```python
from build123d import *

# Parameters (mm, degrees)
BOSS_EXTRUDE1_DEPTH = 1


with BuildPart() as part:
    # Sketch1 → Boss-Extrude1 (new body)
    with BuildSketch(Plane.XY):
        with BuildLine():
            Line((-72.995, -45.925), (-72.995, 45.925))
            ThreePointArc((-72.995, 45.925), (-71.676980515, 49.106980515), (-68.495, 50.425))
            Line((-68.495, 50.425), (61.423932188, 50.425))
            ThreePointArc((61.423932188, 50.425), (63.146007634, 50.082457896), (64.605912703, 49.106980515))
            Line((64.605912703, 49.106980515), (71.676980515, 42.035912703))
            ThreePointArc((71.676980515, 42.035912703), (72.652457896, 40.576007634), (72.995, 38.853932188))
            Line((72.995, 38.853932188), (72.995, -38.853932188))
            ThreePointArc((72.995, -38.853932188), (72.652457896, -40.576007634), (71.676980515, -42.035912703))
            Line((71.676980515, -42.035912703), (64.605912703, -49.106980515))
            ThreePointArc((64.605912703, -49.106980515), (63.146007634, -50.082457896), (61.423932188, -50.425))
            Line((61.423932188, -50.425), (-68.495, -50.425))
            ThreePointArc((-68.495, -50.425), (-71.676980515, -49.106980515), (-72.995, -45.925))
        make_face()
        with BuildLine():
            Line((-71.995, 45.925), (-71.995, -45.925))
            ThreePointArc((-71.995, -45.925), (-70.969873734, -48.399873734), (-68.495, -49.425))
            Line((-68.495, -49.425), (61.423932188, -49.425))
            ThreePointArc((61.423932188, -49.425), (62.763324201, -49.158578364), (63.898805922, -48.399873734))
            Line((63.898805922, -48.399873734), (70.969873734, -41.328805922))
            ThreePointArc((70.969873734, -41.328805922), (71.728578364, -40.193324201), (71.995, -38.853932188))
            Line((71.995, -38.853932188), (71.995, 38.853932188))
            ThreePointArc((71.995, 38.853932188), (71.728578364, 40.193324201), (70.969873734, 41.328805922))
            Line((70.969873734, 41.328805922), (63.898805922, 48.399873734))
            ThreePointArc((63.898805922, 48.399873734), (62.763324201, 49.158578364), (61.423932188, 49.425))
            Line((61.423932188, 49.425), (-68.495, 49.425))
            ThreePointArc((-68.495, 49.425), (-70.969873734, 48.399873734), (-71.995, 45.925))
        make_face(mode=Mode.SUBTRACT)
    extrude(amount=BOSS_EXTRUDE1_DEPTH)


solid = part.part
```
Work out the finished part from the listing and answer in its coordinate system (mm). A direction names the side the tool comes from. Round coordinates to 2 decimals unless told otherwise and drop trailing zeros. Write each loop counter-clockwise with the first axis right and the second up, starting at its lowest first coordinate (ties: lowest second). Pieces come first, ordered by that corner, then holes.
1) A cutting plane is placed at B-B on x = -37. Determine the outline of the cut face in (y, z) (3 decimals), and give its area (3 significant figures).
2) A cutting plane is placed at A-A on y = 30.5. Determine the outline of the cut face in (x, z) (3 decimals).
3) Consider probe 1 along Y at (x, z) = (-44.5, 0.9) (3 decimals); probe 2 along X at (y, z) = (-15, 0.9) (3 decimals); probe 3 along X at (y, z) = (-43, 0.75) (3 decimals). Determine where each line is inside the solid, lowest interval first.
4) Determine the mould class of faces 3 (the face through (-71.712, 49.072, 0.493)), 4 (the face through (68.191, -45.522, 0.493)), 5 (the face through (67.5, 44.8, 0.5)) for opening direction X: pulls with the +X half, pulls with the -X half, needs draft (parallel to the pull), parting line crosses it, or undercut.
5) A cutting plane is placed at C-C on z = 0.75. Determine the outline of the cut face in (x, y) (3 decimals).
6) Which of the six approach directions +Z, -Z, +X, -X, +Y, -Y give full straight-line access (tool end or side, diameter ignored) to faces 1 (the face through (68.092, 45.621, 0.493)), 2 (the face through (-70.94, 48.43, 0.49))?
Entries:
1. outline: (-50.425, 0) - (-49.425, 0) - (-49.425, 1) - (-50.425, 1) - close; (49.425, 0) - (50.425, 0) - (50.425, 1) - (49.425, 1) - close
1. area: 2.00 mm2
2. outline: (-72.995, 0) - (-71.995, 0) - (-71.995, 1) - (-72.995, 1) - close; (71.995, 0) - (72.995, 0) - (72.995, 1) - (71.995, 1) - close
3. probe 1: y = -50.425 to -49.425, 49.425 to 50.425
3. probe 2: x = -72.995 to -71.995, 71.995 to 72.995
3. probe 3: x = -72.995 to -71.995, 69.299 to 70.713
4. face 3: pulls with the -X half
4. face 4: pulls with the +X half
4. face 5: undercut
5. outline: (-72.995, -45.925) arc R4.5 ccw to (-68.495, -50.425) - (61.424, -50.425) arc R4.5 ccw to (64.606, -49.107) - (71.677, -42.036) arc R4.5 ccw to (72.995, -38.854) - (72.995, 38.854) arc R4.5 ccw to (71.677, 42.036) - (64.606, 49.107) arc R4.5 ccw to (61.424, 50.425) - (-68.495, 50.425) arc R4.5 ccw to (-72.995, 45.925) - close; hole (-71.995, -45.925) arc R3.5 ccw to (-68.495, -49.425) - (61.424, -49.425) arc R3.5 ccw to (63.899, -48.4) - (70.97, -41.329) arc R3.5 ccw to (71.995, -38.854) - (71.995, 38.854) arc R3.5 ccw to (70.97, 41.329) - (63.899, 48.4) arc R3.5 ccw to (61.424, 49.425) - (-68.495, 49.425) arc R3.5 ccw to (-71.995, 45.925) - close
6. face 1: +Z, -Z, +X, +Y
6. face 2: +Z, -Z
